Work out the finished part from the listing and answer in its coordinate system (mm). Coordinates: 2 decimals unless noted, no trailing zeros. Loops run counter-clockwise (first coordinate to the right, second up) from the corner with the lowest first, then second, coordinate; pieces in that order, holes last. Notation, with made-up numbers: (53, -14.75) -> (88, -14.75) arc R26 cw to (88, 2.25) -> close; hole circle Ø5 at (4.5, 30.25). An arc over 180 degrees is marked (long way). Use a Markdown table: item, result.
from build123d import *

# Parameters (mm, degrees)
SKETCH_1_R      = 1
EXTRUDE_1_DEPTH = 1.5


with BuildPart() as part:
    # 草图1 → 凸台-拉伸1 (new, symmetric)
    with BuildSketch(Plane.XY):
        with BuildLine():
            Line((0, 2), (40, 2))
            ThreePointArc((40, 2), (42, 0), (40, -2))
            Line((40, -2), (0, -2))
            ThreePointArc((0, -2), (-2, 0), (0, 2))
        make_face()
        Circle(SKETCH_1_R, mode=Mode.SUBTRACT)
    extrude(amount=EXTRUDE_1_DEPTH, both=True)


solid = part.part
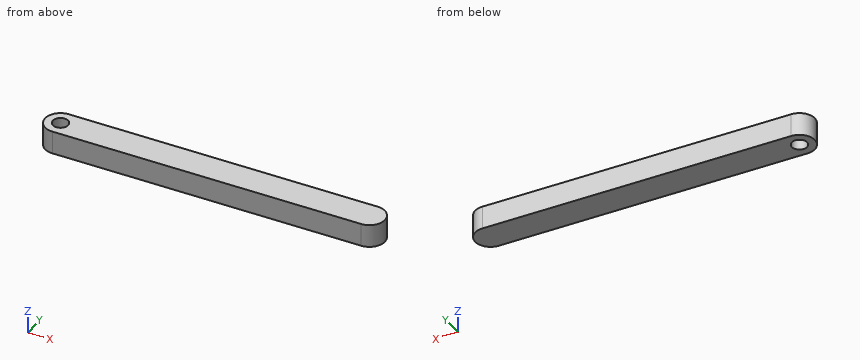
Q1. Consider line 1 (X direction, y = -0.05, z = 1.3); line 2 (Y direction, x = 0, z = -0.15); line 3 (X direction, y = -0.55, z = -0.15). Determine where each line is inside the solid, lowest interval first. Write a range as [from, to].
Solved:
| item | result |
|---|---|
| line 1 | [-2, -1], [1, 42] |
| line 2 | [-2, -1], [1, 2] |
| line 3 | [-1.92, -0.84], [0.84, 41.92] |
Q2. Section A-A on y = 0 is taken. Determine the outline of the cut face in (x, z).
Solved:
| item | result |
|---|---|
| outline | (-2, -1.5) -> (-1, -1.5) -> (-1, 1.5) -> (-2, 1.5) -> close; (1, -1.5) -> (42, -1.5) -> (42, 1.5) -> (1, 1.5) -> close |
Q3. Section B-B on z = 0.15 is taken. Determine the outline of the cut face in (x, y).
Solved:
| item | result |
|---|---|
| outline | (0, -2) -> (40, -2) arc R2 ccw to (40, 2) -> (0, 2) arc R2 ccw to start; hole circle Ø2 at (0, 0) |
